Answer from the drawing. Dimensions are ordinates in mm from the lowest x, y and z of the part. Give positions to 0.01 mm unless a question says otherwise; leave off trailing zeros. Write each loop counter-clockwise with the first axis right and the second up, starting at its lowest first coordinate (ties: lowest second). Pieces come first, ordered by that corner, then holes. Notation, with made-up numbers: M -21,44 L 10,44 A29 cw 10,74 Z; hole C -31,-29.75 d5. An arc over 180 degrees is marked long. Put each result on its own line as item: value.
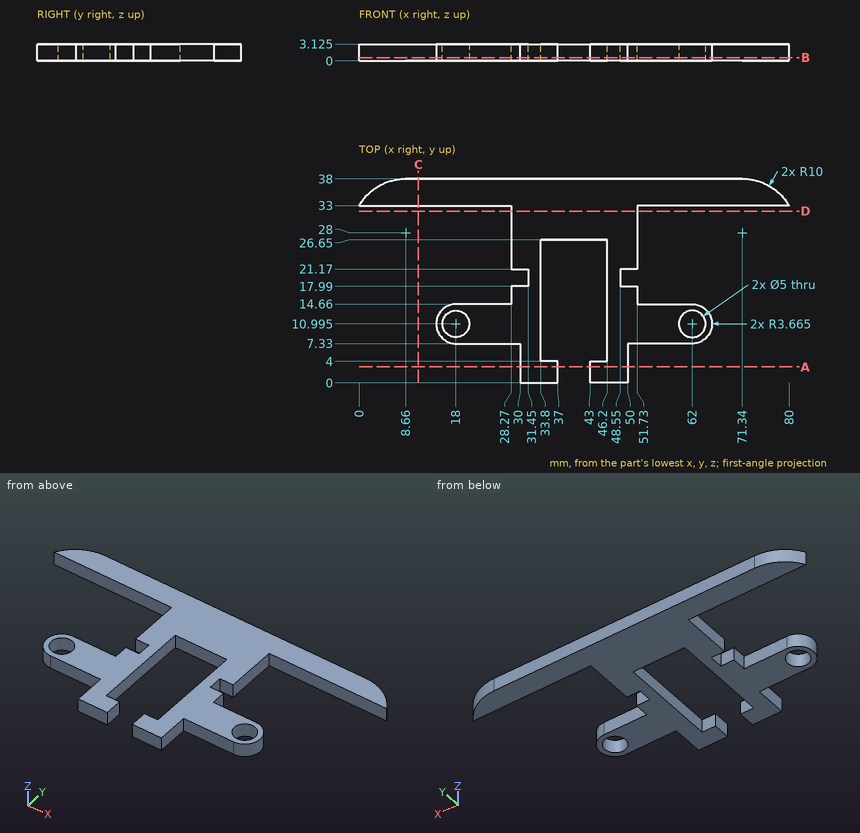
(1) Given pin 1 Ø0.9 at (x, z) = (66.5, 1.5) entering from -Y; pin 2 Ø1.6 at (x, z) = (38.5, 1) entering from -Y; pin 3 Ø1.6 at (y, z) = (27.5, 1.5) entering from -X, each flat-ended and moving along its own axis, determine where each tip first touches the part or whether it passes through.
Result:
pin 1: stops at y = 33
pin 2: stops at y = 26.65
pin 3: stops at x = 28.27
(2) Section B-B on z = 0.6 is taken. Give the number of separate pieces and of enclosed holes in the cut face, and give its area (3 significant figures).
Result:
separate pieces: 1
enclosed holes: 2
area: 952 mm²
(3) Straight lines are drawn through the part: line 1 along Y through (x, z) = (18, 2.1) (1 decimal); line 2 along X through (y, z) = (12, 2.9) (1 decimal); line 3 along X through (y, z) = (21, 2). For each, find the intervals that lie inside material, in ascending order. Write a range as from..to.
Result:
line 1: y = 7.3..8.5, 13.5..14.7, 33..38
line 2: x = 14.5..15.7, 20.3..33.8, 46.2..59.7, 64.3..65.5
line 3: x = 31.45..33.8, 46.2..48.55
(4) Section A-A on y = 3 is taken. Determine the outline of the cut face in (x, z) (1 decimal).
Result:
outline: M 30,0 L 37,0 L 37,3.1 L 30,3.1 Z; M 43,0 L 50,0 L 50,3.1 L 43,3.1 Z
(5) Section D-D on y = 32 is taken. Determine the outline of the cut face in (x, z) (1 decimal), and give its area (3 significant figures).
Result:
outline: M 28.3,0 L 51.7,0 L 51.7,3.1 L 28.3,3.1 Z
area: 73.3 mm²
(6) Section C-C on x = 11 is taken. Determine the outline of the cut face in (y, z) (1 decimal).
Result:
outline: M 33,0 L 38,0 L 38,3.1 L 33,3.1 Z
